from build123d import *

# Parameters (mm, degrees)
SKETCH1_R                = 1
BOSS_EXTRUDE1_DEPTH      = 5.75
BOSS_EXTRUDE2_DEPTH      = 6.5
BOSS_EXTRUDE2_DEPTH_BACK = 3.5
SKETCH3_W                = 6
SKETCH3_H                = 2.75
BOSS_EXTRUDE3_DEPTH      = 9.5
BOSS_EXTRUDE3_DEPTH_BACK = 3.5
SKETCH3_5_R              = 8
SKETCH3_5_R_2            = 6
CUT_EXTRUDE1_DEPTH       = 36.96265424
CUT_EXTRUDE1_DEPTH_BACK  = 36.96265424
SKETCH3_6_R              = 6
SKETCH3_6_R_2            = 1.5
CUT_EXTRUDE3_START       = 1.5
SKETCH3_8_R              = 1.5
CUT_EXTRUDE3_DEPTH       = 2
FILLET1_R                = 3
CHAMFER1_SIZE            = 2
BOSS_EXTRUDE4_DEPTH      = 3.5
CUT_EXTRUDE5_DEPTH       = 4.494021888
CUT_EXTRUDE6_DEPTH       = 5.692616578
FILLET2_R                = 0.5
CUT_EXTRUDE8_DEPTH       = 57.979942817
CUT_EXTRUDE8_DEPTH_BACK  = 10
SKETCH11_R               = 1.5
LPATTERN1_COUNT          = 2
LPATTERN1_PITCH          = 5
SKETCH14_R               = 1
BOSS_EXTRUDE5_DEPTH      = 11.5


with BuildPart() as part:
    # Sketch1 → Boss-Extrude1 (new, symmetric)
    with BuildSketch(Plane(origin=(0, 0, 0), x_dir=(0, 0, -1), z_dir=(1, 0, 0))):
        with BuildLine():
            Line((-3.5, 19), (3.5, 19))
            Line((3.5, 19), (3.5, -23.51))
            ThreePointArc((3.5, -23.51), (0, -27.01), (-3.5, -23.51))
            Line((-3.5, -23.51), (-3.5, 19))
        make_face()
        with Locations((0.25, -23.76)):
            Circle(SKETCH1_R, mode=Mode.SUBTRACT)
    extrude(amount=BOSS_EXTRUDE1_DEPTH, both=True)



with BuildPart() as body_2:
    # Sketch3 → Boss-Extrude2 (new, two sides: drawn at the far end of the back side and taken through both)
    with BuildSketch(Plane.XY.offset(-BOSS_EXTRUDE2_DEPTH_BACK)):
        with BuildLine():
            ThreePointArc((-6, 24.291502622), (0, 27), (6, 24.291502622))
            Line((6, 24.291502622), (6, 31.641502622))
            ThreePointArc((6, 31.641502622), (0, 33.75), (-6, 31.641502622))
            Line((-6, 31.641502622), (-6, 24.291502622))
        make_face()
        with Locations((0, 29.375)):
            Rectangle(SKETCH3_W, SKETCH3_H, mode=Mode.SUBTRACT)
    extrude(amount=BOSS_EXTRUDE2_DEPTH + BOSS_EXTRUDE2_DEPTH_BACK)


with BuildPart() as part_1:
    add(part.part)

    add(body_2.part)  # Boss-Extrude3 merges body 2
    # Sketch3<5> → Boss-Extrude3 (add, two sides: drawn at the far end of the back side and taken through both)
    with BuildSketch(Plane.XY.offset(-BOSS_EXTRUDE3_DEPTH_BACK)):
        with Locations((0, 19)):
            Circle(SKETCH3_5_R)
        with Locations((0, 19)):
            Circle(SKETCH3_5_R_2, mode=Mode.SUBTRACT)
    extrude(amount=BOSS_EXTRUDE3_DEPTH + BOSS_EXTRUDE3_DEPTH_BACK)

    # Sketch3<6> → Cut-Extrude1 (cut, two sides: drawn at the far end of the back side and taken through both)
    with BuildSketch(Plane.XY.offset(-CUT_EXTRUDE1_DEPTH_BACK)):
        with Locations((0, 19)):
            Circle(SKETCH3_6_R)
        with Locations((0, -8.5)):
            Circle(SKETCH3_6_R_2)
    extrude(amount=CUT_EXTRUDE1_DEPTH + CUT_EXTRUDE1_DEPTH_BACK, mode=Mode.SUBTRACT)

    # Sketch3<8> → Cut-Extrude3 (cut)
    with BuildSketch(Plane.XY.offset(CUT_EXTRUDE3_START)):
        Polygon((4, -14.65), (4, 11), (0, 11), (-4, 11), (-4, -14.65), align=None)
        with Locations((0, -8.5)):
            Circle(SKETCH3_8_R, mode=Mode.SUBTRACT)
    extrude(amount=CUT_EXTRUDE3_DEPTH, mode=Mode.SUBTRACT)

    # Fillet1
    fillet1_edges = [part_1.edges().sort_by_distance(p)[0] for p in [
        (4, 11, 2.5),
        (-4, 11, 2.5),
    ]]
    fillet(fillet1_edges, radius=FILLET1_R)

    # Chamfer1
    chamfer1_edges = [part_1.edges().sort_by_distance(p)[0] for p in [
        (0, -14.65, 3.5),
    ]]
    chamfer(chamfer1_edges, length=CHAMFER1_SIZE - 0.0001)  # a hair under: the kernel refuses the full size

    # Sketch6 → Boss-Extrude4 (add, symmetric)
    with BuildSketch(Plane.XY):
        with BuildLine():
            Line((-5.75, -20), (-5.75, 13.437851135))
            ThreePointArc((-5.75, 13.437851135), (-7.539998072, 16.32634537), (-7.969557585, 19.697245942))
            Line((-7.969557585, 19.697245942), (-11.442616578, -20))
            Line((-11.442616578, -20), (-5.75, -20))
        make_face()
        with BuildLine():
            ThreePointArc((5.75, 13.437851135), (7.539998072, 16.32634537), (7.969557585, 19.697245942))
            Line((7.969557585, 19.697245942), (10.244021888, -6.3))
            Line((10.244021888, -6.3), (5.75, -6.3))
            Line((5.75, -6.3), (5.75, 13.437851135))
        make_face()
    extrude(amount=BOSS_EXTRUDE4_DEPTH, both=True)

    # Sketch8 → Cut-Extrude5 (cut)
    with BuildSketch(Plane(origin=(10.244021888, 0, 0), x_dir=(0, 0, -1), z_dir=(1, 0, 0))):
        Polygon((-3.5, -6.3), (3.5, -2.258548116), (3.5, -6.3), align=None)
    extrude(amount=-CUT_EXTRUDE5_DEPTH, mode=Mode.SUBTRACT)

    # Sketch9 → Cut-Extrude6 (cut)
    with BuildSketch(Plane.ZY.offset(11.442616578)):
        Polygon((-3.5, -20), (-3.5, -16.735846393), (3.5, -20), align=None)
    extrude(amount=-CUT_EXTRUDE6_DEPTH, mode=Mode.SUBTRACT)

    # Fillet2
    fillet2_edges = [part_1.edges().sort_by_distance(p)[0] for p in [
        (-8.596308289, -20, 3.5),
        (7.997010944, -6.3, 3.5),
        (7.820220332, -2.258548116, -3.5),
        (-8.453520071, -16.735846393, -3.5),
    ]]
    fillet(fillet2_edges, radius=FILLET2_R)

    # Sketch11 → Cut-Extrude8 (cut, two sides: drawn at the far end of the back side and taken through both)
    with BuildSketch(Plane(origin=(0, 28, 0), x_dir=(1, 0, 0), z_dir=(0, 1, 0)).offset(-CUT_EXTRUDE8_DEPTH_BACK)):
        with Locations(Location((0, -1.5, 0), (0, 0, 270))):
            Circle(SKETCH11_R)
    extrude(amount=CUT_EXTRUDE8_DEPTH + CUT_EXTRUDE8_DEPTH_BACK, mode=Mode.SUBTRACT)

    # Sketch13 → M3 Tapped Hole1 (revolve, cut)
    with BuildSketch(Plane(origin=(-9.619215273, 0.841572288, 0), x_dir=(-0.08715574274765137, -0.9961946980917462, 0), z_dir=(0, 0, 1))):
        Polygon((0, 0), (0, 7.851075774), (1.25, 7.1), (1.25, 0.275), (1.525, 0), align=None)
    m3_tapped_hole1 = revolve(axis=Axis((-15.945051605, 1.395011255, 0), (0.996194698091746, -0.08715574274765134, 0)), mode=Mode.SUBTRACT)

    # LPattern1: M3 Tapped Hole1 ×2
    with Locations(*[Vector(-0.08715574274765112, -0.9961946980917462, 0) * (i * LPATTERN1_PITCH) for i in range(1, LPATTERN1_COUNT)]):
        add(m3_tapped_hole1, mode=Mode.SUBTRACT)

    # Sketch14 → Boss-Extrude5 (add)
    with BuildSketch(Plane.ZY.offset(5.75)):
        with Locations((-0.25, -23.76)):
            Circle(SKETCH14_R)
    extrude(amount=-BOSS_EXTRUDE5_DEPTH)

    # Sketch16 → M3 Tapped Hole2 (revolve, cut)
    with BuildSketch(Plane(origin=(-5.75, -23.76, -0.25), x_dir=(0, 0, 1), z_dir=(0, 1, 0))):
        Polygon((0, 0), (0, 11.5), (1.525, 11.5), (1.25, 11.225), (1.25, 0.275), (1.525, 0), align=None)
    revolve(axis=Axis((-12.1, -23.76, -0.25), (1, 0, 0)), mode=Mode.SUBTRACT)


solid = part_1.part
For this review, take the finished solid that the model builds, in its own axes (mm). A direction names the side the tool comes from. Give positions to 0.01 mm unless a question says otherwise; leave off trailing zeros. Loops run counter-clockwise (first coordinate to the right, second up) from the corner with the lowest first, then second, coordinate; pieces in that order, holes last. Notation, with made-up numbers: M -6.5,6.25 L 10.5,6.25 A32 cw 10.5,36.25 Z; hole C 85.25,54.25 d8. An arc over 180 degrees is marked long. Put each result on its own line as item: value. Start each with the question number.
(1) Add section B-B, the plane y = 5. Write out the cut boundary in (x, z).
(2) Add section A-A, the plane y = -8.5. Write out the cut boundary in (x, z), then the cut area to 3 significant figures.
(3) For pin 1 (2 mm diameter, centred on y = 27, z = 2.5, fed in from +X); pin 2 (6 mm diameter, centred on x = 7.5, z = 7.5, fed in from +Y); pin 3 (5.5 mm diameter, centred on y = -19.5, z = -1, fed in from -X); pin 4 (1.5 mm diameter, centred on y = -23.76, z = -0.25, fed in from +X), all flat-tipped, find the tip position at first contact; note any pin that passes through.
(4) Wall thickness on L1, parallel to Z at x = 0, y = 33; L2, parallel to Y at x = 3.5, z = 3; L3, parallel to Y at x = 0, z = 5.5: over which ranges is each line inside the solid? List them lowest first.
(5) Machinability: for faces 1 (the cylindrical face through (7.39, 15.94, 5.8)), 2 (the flat face through (-8.62, -18.25, -0.25)), 3 (the conical face through (-1.91, 0.34, 0.13)), 4 (the flat face through (9.075, 7.061, 0.049)), 5 (the flat face through (-3, 29, 1)), which of the approach directions +Z, -Z, +X, -X, +Y, -Y give a long, thin tool a straight path to every point of the face, cutting with its end or side? Answer none if there is none.
(6) The part is to be moulded in two halves that separate along Y. For faces 6 (the flat face through (0, -2, 1.5)), 7 (the flat face through (-1, 6, -3.5)), 8 (the cylindrical face through (1.52, 33.63, 2.54)), 9 (the flat face through (8.01, -4.16, -0.21)), say which applies: +Y half, -Y half, draft (parallel to the pull), parting line (faces both ways), or undercut.
Result:
1. outline: M -9.26,-3.5 L 9.26,-3.5 L 9.26,3.5 L 4,3.5 L 4,1.5 L -4,1.5 L -4,3.5 L -9.26,3.5 Z
2. outline: M -10.44,-3.5 L -1.5,-3.5 L -1.5,1.5 L -4,1.5 L -4,3.5 L -10.44,3.5 Z; M 1.5,-3.5 L 5.75,-3.5 L 5.75,3.5 L 4,3.5 L 4,1.5 L 1.5,1.5 Z
2. area: 82.3 mm^2
3. pin 1: stops at x = 6
3. pin 2: stops at y = 32.54
3. pin 3: stops at x = -11.37
3. pin 4: passes through
4. L1: z = -3.5 to 0, 3 to 6.5
4. L2: y = -25.31 to -16.15, 9.66 to 14.13, 23.87 to 33.09
4. L3: y = 11 to 13, 25 to 28, 30.75 to 33.75
5. face 1: +Z
5. face 2: -Z, -X, -Y
5. face 3: none
5. face 4: +Z, -Z, +X, +Y
5. face 5: +Z, -Z
6. face 6: undercut
6. face 7: draft
6. face 8: +Y half
6. face 9: -Y half
